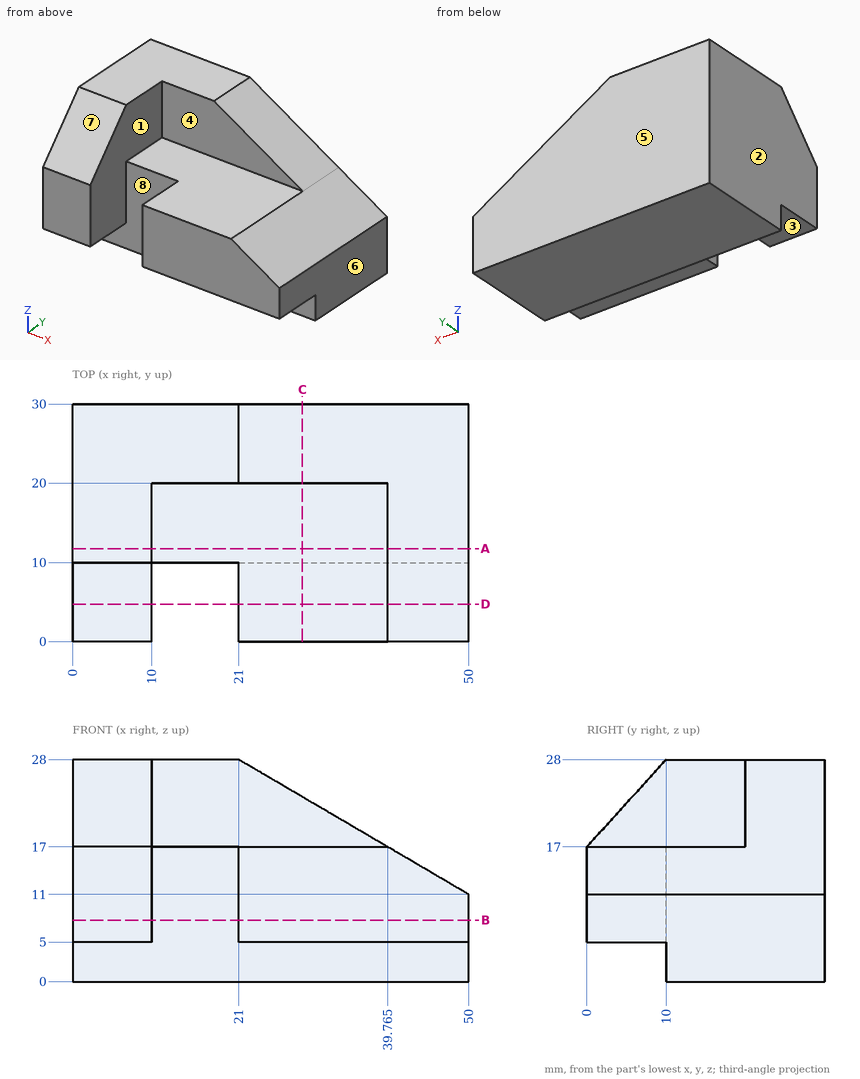
Geometry check sheet. Reference: drawing and pictorial views, mm from the part's lowest x, y, z. A direction names the side the tool comes from. Coordinates: 2 decimals unless noted, no trailing zeros. Order: outer loops, then holes, each group sorted by start corner. A loop starts at its lowest first (then second) coordinate and runs counter-clockwise, first axis right, second up. Notation, with made-up numbers: (67, 2.5) - (79, 2.5) arc R21 cw to (79, 9.5) - close; hole circle Ø9 at (73.5, 17). An arc over 180 degrees is marked (long way). Answer in a Markdown table with one row per item. Add a question column.
1) Gauge pin test, flat ends, axial feed: P1, Ø5, axis at x = 4, y = 4, coming from the -Z side; P2, Ø5, axis at x = 34, y = 16, coming from the +Z side; P3, Ø6, axis at y = 13.5, z = 20.5, coming from the +X side. Record the tip position at first contact, or that the pin passes through.
2) Cross-section at A-A, the plane y = 11.75. Record the cut outline in (x, z) (1 decimal).
3) Cross-section at D-D, the plane y = 4.75. Record the cut outline in (x, z) (1 decimal).
4) Cross-section at B-B, the plane z = 7.75. Record the cut outline in (x, y).
5) Release check for a two-part mould opening along X. For the marked faces 6, 7 and 8 record: +X half, -X half, draft (parallel to the pull), parting line (faces both ways), or undercut.
6) Material ranges on line 1 along Y through (x, z) = (22, 17.5); line 2 along X through (y, z) = (4.25, 19.5); line 3 along Y through (x, z) = (7, 4.5), recorded low to high. Write a range as [from, to].
7) Set-up check for the marked faces 1, 2, 3, 4 and 5: record each of +Z, -Z, +X, -X, +Y, -Y from which the full face is reachable in a straight line by a thin tool's end or side.
8) Cross-section at C-C, the plane x = 29. Record the cut outline in (y, z).
Check result:
| question | item | result |
|---|---|---|
| 1 | P1 | stops at z = 5 |
| 1 | P2 | stops at z = 17 |
| 1 | P3 | stops at x = 10 |
| 2 | outline | (0, 0) - (50, 0) - (50, 11) - (39.8, 17) - (10, 17) - (10, 28) - (0, 28) - close |
| 3 | outline | (0, 5) - (10, 5) - (10, 22.2) - (0, 22.2) - close; (21, 5) - (50, 5) - (50, 11) - (39.8, 17) - (21, 17) - close |
| 4 | outline | (0, 0) - (10, 0) - (10, 10) - (21, 10) - (21, 0) - (50, 0) - (50, 30) - (0, 30) - close |
| 5 | face 6 | +X half |
| 5 | face 7 | draft |
| 5 | face 8 | undercut |
| 6 | line 1 | y = [20, 30] |
| 6 | line 2 | x = [0, 10] |
| 6 | line 3 | y = [10, 30] |
| 7 | face 1 | +Z, -Y |
| 7 | face 2 | +Z, -Z, -X, +Y, -Y |
| 7 | face 3 | -Z, +X, -X, -Y |
| 7 | face 4 | +Z, +X, -Y |
| 7 | face 5 | +Z, -Z, +X, -X, +Y |
| 8 | outline | (0, 5) - (10, 5) - (10, 0) - (30, 0) - (30, 23.31) - (20, 23.31) - (20, 17) - (0, 17) - close |
